The listing builds one solid part. Answer for the finished solid, in the listing's coordinates (mm). A direction names the side the tool comes from. Coordinates: 2 decimals unless noted, no trailing zeros. Write each loop counter-clockwise with the first axis right and the second up, starting at its lowest first coordinate (ties: lowest second). Pieces come first, ordered by that corner, then holes.
Autodesk Inventor part; units mm, degrees
ref_plane "YZ Plane" through (0, 0, 0) normal (1, 0, 0) x (0, 1, 0)
ref_plane "XZ Plane" through (0, 0, 0) normal (0, 1, 0) x (-1, 0, 0)
ref_plane "XY Plane" through (0, 0, 0) normal (0, 0, 1) x (1, 0, 0)
sketch "Sketch1" plane through (0, 0, 0) normal (0, 1, 0) x (-1, 0, 0)
  line L0 (6.35, 3.6662) -> (6.35, -3.6662)
  line L1 (6.35, -3.6662) -> (0, -7.3323)
  line L2 (0, -7.3323) -> (-6.35, -3.6662)
  line L3 (-6.35, -3.6662) -> (-6.35, 3.6662)
  line L4 (-6.35, 3.6662) -> (0, 7.3323)
  line L5 (0, 7.3323) -> (6.35, 3.6662)
  point P0 (0, 0)
  point P1 (0, 0)
  dimension "d0" = 12.7
extrude "Extrusion1" add sketch "Sketch1" along normal blind 315.3029
sketch "Sketch2" plane through (0, 315.3029, 0) normal (0, 1, 0) x (1, 0, 0)
  circle A0 centre (0, 0) radius 2.5527
  dimension "d3" = 5.1054
extrude "Extrusion2" cut sketch "Sketch2" against normal blind 50.8
sketch "Sketch3" plane through (0, 0, 0) normal (0, -1, 0) x (1, 0, 0)
  circle A0 centre (0, 0) radius 2.5527
  dimension "d6" = 5.1054
extrude "Extrusion3" cut sketch "Sketch3" against normal blind 50.8
thread "Thread1"
properties part number "CORL_010_DropGearShaft" material "Aluminum 6061"
Q1. Which of the six approach directions +Z, -Z, +X, -X, +Y, -Y give full straight-line access (tool end or side, diameter ignored) to faces 4 (the face through (0, 264.503, 0)), 5 (the face through (0, 50.8, 0)), 6 (the face through (6.35, 155, 0))?
Answers below:
face 4: +Y
face 5: -Y
face 6: +Z, -Z, +X, +Y, -Y
Q2. Given pin 1 (3 mm diameter, centred on x = 0, z = 0, fed in from -Y); pin 2 (1.5 mm diameter, centred on x = -1, z = 0.5, fed in from +Y); pin 3 (2 mm diameter, centred on x = -2.5, y = 47.5, fed in from +Z), each flat-ended and moving along its own axis, determine where each tip first touches the part or whether it passes through.
Answers below:
pin 1: stops at y = 50.8
pin 2: stops at y = 264.5
pin 3: stops at z = 6.47
Q3. The part is cut by section B-B, the plane z = 0. Write down the section's boundary in (x, y).
Answers below:
outline: (-6.35, 0) - (-2.55, 0) - (-2.55, 50.8) - (2.55, 50.8) - (2.55, 0) - (6.35, 0) - (6.35, 315.3) - (2.55, 315.3) - (2.55, 264.5) - (-2.55, 264.5) - (-2.55, 315.3) - (-6.35, 315.3) - close
Q4. Determine the mould class of faces 1 (the face through (0, 0, -3)), 2 (the face through (2.435, 25.044, 0.767)), 3 (the face through (3.219, 155.444, 5.474)) for opening direction X: released by +X, released by -X, zero draft, split by the parting line, or undercut.
Answers below:
face 1: zero draft
face 2: undercut
face 3: released by +X
Q5. The part is cut by section A-A, the plane y = 293. Write down the section's boundary in (x, z).
Answers below:
outline: (-6.35, -3.67) - (0, -7.33) - (6.35, -3.67) - (6.35, 3.67) - (0, 7.33) - (-6.35, 3.67) - close; hole circle Ø5.11 at (0, 0)
Q6. Find the intervals of material crossed by probe 1 along Z at (x, y) = (0, 26); probe 2 along X at (y, z) = (280.5, 0); probe 3 along Y at (x, z) = (0, 1.5), in increasing order.
Answers below:
probe 1: z = -7.33 to -2.55, 2.55 to 7.33
probe 2: x = -6.35 to -2.55, 2.55 to 6.35
probe 3: y = 50.8 to 264.5
Q7. The part is cut by section C-C, the plane y = 241. Write down the section's boundary in (x, z).
Answers below:
outline: (-6.35, -3.67) - (0, -7.33) - (6.35, -3.67) - (6.35, 3.67) - (0, 7.33) - (-6.35, 3.67) - close
